For this review, take the finished solid that the model builds, in its own axes (mm). Face numbers are marked on the shaded views. A direction names the side the tool comes from. Round coordinates to 2 decimals unless told otherwise and drop trailing zeros. Write each loop counter-clockwise with the first axis right and the second up, starting at its lowest first coordinate (ties: lowest second). Pieces come first, ordered by that corner, then holes.
from build123d import *

# Parameters (mm, degrees)
SKETCH1_W                  = 25.4
SKETCH1_H                  = 25.4
BOSS_EXTRUDE1_DEPTH        = 6.35
SKETCH2_W                  = 17.78
SKETCH2_H                  = 17.78
CUT_EXTRUDE1_DEPTH         = 3.0226
FILLET1_R                  = 4.7625
F_10_CLEARANCE_HOLE1_D     = 5.1054
F_10_CLEARANCE_HOLE1_DEPTH = 10.668
F_10_CLEARANCE_HOLE1_TIP   = 1.533816902
FILLET2_R                  = 0.78


with BuildPart() as part:
    # Sketch1 → Boss-Extrude1 (new body)
    with BuildSketch(Plane(origin=(0, 0, 0), x_dir=(1, 0, 0), z_dir=(0, 1, 0))):
        Rectangle(SKETCH1_W, SKETCH1_H)
    extrude(amount=BOSS_EXTRUDE1_DEPTH)

    # Sketch2 → Cut-Extrude1 (cut)
    with BuildSketch(Plane.XZ):
        with Locations((-3.81, 3.81)):
            Rectangle(SKETCH2_W, SKETCH2_H)
    extrude(amount=-CUT_EXTRUDE1_DEPTH, mode=Mode.SUBTRACT)

    # Fillet1
    fillet1_edges = [part.edges().sort_by_distance(p)[0] for p in [
        (12.7, 3.175, 12.7),
        (-12.7, 4.6863, 12.7),
        (-12.7, 3.175, -12.7),
        (12.7, 3.175, -12.7),
    ]]
    fillet(fillet1_edges, radius=FILLET1_R)

    # #10 Clearance Hole1
    with Locations(Plane(origin=(0, 6.35, 0), x_dir=(1, 0, 0), z_dir=(0, 1, 0))):
        with Locations((7.9375, 7.9375)):
            Hole(F_10_CLEARANCE_HOLE1_D / 2, depth=F_10_CLEARANCE_HOLE1_DEPTH)
            with Locations((0, 0, -(F_10_CLEARANCE_HOLE1_DEPTH + F_10_CLEARANCE_HOLE1_TIP / 2))):  # 118° drill point
                Cone(0, F_10_CLEARANCE_HOLE1_D / 2, F_10_CLEARANCE_HOLE1_TIP, mode=Mode.SUBTRACT)

    # Fillet2
    fillet2_edges = [part.edges().sort_by_distance(p)[0] for p in [
        (0, 6.35, 12.7),
        (-12.7, 6.35, 0),
        (12.7, 6.35, 0),
        (0, 6.35, -12.7),
        (11.305096045, 6.35, 11.305096045),
        (11.305096045, 6.35, -11.305096045),
        (-11.305096045, 6.35, -11.305096045),
        (-11.305096045, 6.35, 11.305096045),
    ]]
    fillet(fillet2_edges, radius=FILLET2_R)


solid = part.part
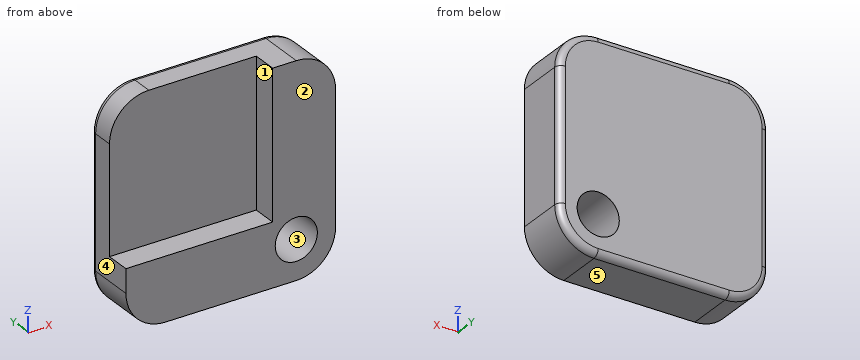
(1) We need section D-D, the plane y = 1.75. Give the boundary of the cut face in (x, z) (1 decimal).
Geometry check:
outline: (-12.7, -7.9) arc R4.8 ccw to (-7.9, -12.7) - (7.9, -12.7) arc R4.8 ccw to (12.7, -7.9) - (12.7, 7.9) arc R4.8 ccw to (7.9, 12.7) - (5.1, 12.7) - (5.1, -5.1) - (-12.7, -5.1) - close; hole circle Ø5.1 at (7.9, -7.9)
(2) We need section B-B, the plane x = -3.25. Give the boundary of the cut face in (y, z), and give its area (3 significant figures).
Geometry check:
outline: (0, -12.7) - (5.57, -12.7) arc R0.78 ccw to (6.35, -11.92) - (6.35, 11.92) arc R0.78 ccw to (5.57, 12.7) - (3.02, 12.7) - (3.02, -5.08) - (0, -5.08) - close
area: 107 mm2
(3) For line 1 along Z through (x, y) = (7.75, 4); line 2 along Z through (x, y) = (-4.5, 2.75); line 3 along X through (y, z) = (2, 8), list the stretches that pass through material, from the lowest coordinate up.
Geometry check:
line 1: z = -12.7 to -10.48, -5.39 to 12.7
line 2: z = -12.7 to -5.08
line 3: x = 5.08 to 12.7
(4) Mouldability with a two-part tool opening along X and no side actions: class the marked faces 3, 4 and 5 as pulls with the +X half, pulls with the -X half, needs draft (parallel to the pull), parting line crosses it, or undercut.
Geometry check:
face 3: undercut
face 4: pulls with the -X half
face 5: needs draft
(5) We need section A-A, the plane y = 3.5. Give the boundary of the cut face in (x, z) (1 decimal), and give its area (3 significant figures).
Geometry check:
outline: (-12.7, -7.9) arc R4.8 ccw to (-7.9, -12.7) - (7.9, -12.7) arc R4.8 ccw to (12.7, -7.9) - (12.7, 7.9) arc R4.8 ccw to (7.9, 12.7) - (-7.9, 12.7) arc R4.8 ccw to (-12.7, 7.9) - close; hole circle Ø5.1 at (7.9, -7.9)
area: 605 mm2
(6) For pin 1 Ø9 at (x, z) = (-1.5, 4.5) entering from -Y; pin 2 Ø1.5 at (x, y) = (-6.5, 1) entering from +Z; pin 3 Ø2.5 at (y, z) = (1.5, 6) entering from -X, all flat-tipped, find the tip position at first contact; note any pin that passes through.
Geometry check:
pin 1: stops at y = 3.02
pin 2: stops at z = -5.08
pin 3: stops at x = 5.08
(7) We need section C-C, the plane z = -7.25. Give the boundary of the cut face in (x, y), and give its area (3 significant figures).
Geometry check:
outline: (-12.7, 0) - (5.48, 0) - (5.48, 6.35) - (-11.92, 6.35) arc R0.78 ccw to (-12.7, 5.57) - close; (10.4, 0) - (12.7, 0) - (12.7, 5.57) arc R0.78 ccw to (11.92, 6.35) - (10.4, 6.35) - close
area: 130 mm2
(8) For the marked faces 1 and 2, list the 3-axis set-ups (+Z, -Z, +X, -X, +Y, -Y) from which the entire face can be reached by the end or side of a thin tool; tool diameter is ignored.
Geometry check:
face 1: +Z, -X, -Y
face 2: +Z, -Z, +X, -X, -Y
